from build123d import *

# Parameters (mm, degrees)
SKETCH_2_W          = 25
SKETCH_2_H          = 25
EXTRUDE_1_DEPTH     = 3
SKETCH_3_R          = 1.5
CUT_EXTRUDE_2_DEPTH = 4
EXTRUDE_START       = -3
SKETCH_4_R          = 10
EXTRUDE_2_DEPTH     = 27
SKETCH_5_R          = 3.05
EXTRUDE_3_DEPTH     = 8
FILLET_3_R          = 1


with BuildPart() as part:
    # 草图2 → 凸台-拉伸1 (new body)
    with BuildSketch(Plane.XY):
        with Locations((12.5, -12.5)):
            Rectangle(SKETCH_2_W, SKETCH_2_H)
    extrude(amount=EXTRUDE_1_DEPTH)

    # 草图3 → 切除-拉伸2 (cut, through all)
    with BuildSketch(Plane(origin=(0, 0, 0), x_dir=(-1, 0, 0), z_dir=(0, 0, -1))):
        with Locations((-22, -3)):
            Circle(SKETCH_3_R)
        with Locations((-3, -3)):
            Circle(SKETCH_3_R)
        with Locations((-3, -22)):
            Circle(SKETCH_3_R)
        with Locations((-22, -22)):
            Circle(SKETCH_3_R)
    extrude(amount=-CUT_EXTRUDE_2_DEPTH, mode=Mode.SUBTRACT)

    # 草图4 → 凸台-拉伸2 (add)
    with BuildSketch(Plane.XY.offset(3).offset(EXTRUDE_START)):
        with Locations((12.5, -12.5)):
            Circle(SKETCH_4_R)
    extrude(amount=-EXTRUDE_2_DEPTH)

    # 草图5 → 凸台-拉伸3 (add)
    with BuildSketch(Plane(origin=(0, 0, -27), x_dir=(-1, 0, 0), z_dir=(0, 0, -1))):
        with Locations((-12.5, -12.5)):
            Circle(SKETCH_5_R)
    extrude(amount=EXTRUDE_3_DEPTH)

    # 圆角3
    fillet_3_edges = [part.edges().sort_by_distance(p)[0] for p in [
        (2.5, -12.5, -27),
        (2.5, -12.5, 0),
    ]]
    fillet(fillet_3_edges, radius=FILLET_3_R)


solid = part.part
Verification items for the finished model (mm, model axes). A direction names the side the tool comes from. Give positions to 0.01 mm unless a question says otherwise; leave off trailing zeros. Order: outer loops, then holes, each group sorted by start corner. A loop starts at its lowest first (then second) coordinate and runs counter-clockwise, first axis right, second up. Notation, with made-up numbers: (-14.5, 22) -> (-9.5, 22) arc R23 cw to (-9.5, 57) -> close; hole circle Ø1 at (53.5, 56). An arc over 180 degrees is marked (long way). Answer as CSV lines item,"result".
Q1. Release check for a two-part mould opening along Y. For faces 3 (the cylindrical face through (23.5, -2.93, 1.48)), 4 (the cylindrical face through (23.11, -20.99, 1.48)), 5 (the flat face through (12, -16, -27)), 6 (the flat face through (12, -25, 1)) record: +Y half, -Y half, draft (parallel to the pull), parting line (faces both ways), or undercut.
Solutions:
face 3,"undercut"
face 4,"undercut"
face 5,"draft"
face 6,"-Y half"
Q2. Sectioned sample at B-B on z = -30. Record the cut outline in (x, y).
Solutions:
outline,"circle Ø6.1 at (12.5, -12.5)"
Q3. Depth check by flat-ended pin: pin 1 (1 mm diameter, centred on y = -6.5, z = -1, fed in from -X); pin 2 (12 mm diameter, centred on x = 4, z = -26.5, fed in from -Y); pin 3 (4 mm diameter, centred on x = 22, y = -3, fed in from -Z); pin 4 (2.5 mm diameter, centred on x = 3, y = -22, fed in from -Z). Enter the tip coordinate at first touch or a pass-through.
Solutions:
pin 1,"stops at x = 4.15"
pin 2,"stops at y = -22.18"
pin 3,"stops at z = 0"
pin 4,"passes through"
Q4. Scan lines: probe 1 along Y at (x, z) = (3, 0.65); probe 2 along X at (y, z) = (-12.25, -29); probe 3 along Z at (x, y) = (10.5, -9.75). Record each from-to range of solid material in increasing order.
Solutions:
probe 1,"y = -25 to -23.5, -20.5 to -4.5, -1.5 to 0"
probe 2,"x = 9.46 to 15.54"
probe 3,"z = -27 to 3"
Q5. Sectioned sample at A-A on x = 12.5. Record the cut outline in (y, z).
Solutions:
outline,"(-25, 0) -> (-23.5, 0) arc R1 cw to (-22.5, -1) -> (-22.5, -26) arc R1 ccw to (-21.5, -27) -> (-15.55, -27) -> (-15.55, -35) -> (-9.45, -35) -> (-9.45, -27) -> (-3.5, -27) arc R1 ccw to (-2.5, -26) -> (-2.5, -1) arc R1 cw to (-1.5, 0) -> (0, 0) -> (0, 3) -> (-25, 3) -> close"
Q6. Sectioned sample at C-C on y = -22. Count the separate pieces of the cut face and the enclosed holes in it, plus the area to 3 significant figures.
Solutions:
separate pieces,"3"
enclosed holes,"0"
area,"225 mm²"
Q7. Access from +Z, -Z, +X, -X, +Y, -Y to the whole of each face (thin tool, end or side, straight path). Record for faces 1 (the flat face through (12, -1, 0)), 2 (the flat face through (12, 0, 1)).
Solutions:
face 1,"-Z"
face 2,"+Z, -Z, +X, -X, +Y"
